Geometry: see drawing. Coordinates: mm, zero at the bounding-box minimum. Coordinates: 2 decimals unless noted, no trailing zeros. Write each loop counter-clockwise with the first axis right and the second up, starting at its lowest first coordinate (ties: lowest second). Pieces come first, ordered by that corner, then holes.
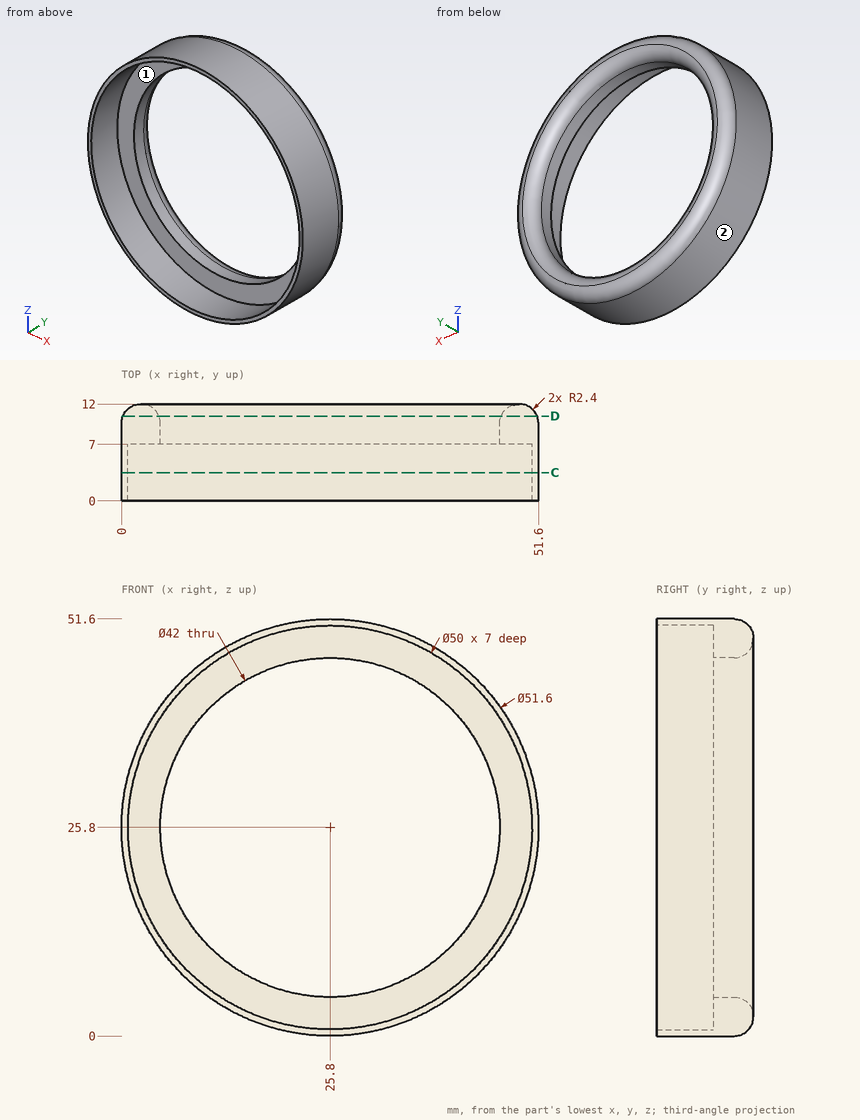
Item 1: Pull-direction query (Z, two-part tool) for the marked faces 1 and 2; classes: released by +Z, released by -Z, zero draft, split by the parting line, or undercut.
Derived:
face 1: undercut
face 2: split by the parting line
Item 2: Material intervals for probe 1 along X at (y, z) = (3.5, 25.8); probe 2 along X at (y, z) = (9, 25.8); probe 3 along Z at (x, y) = (7, 7.5), sorted ascending.
Derived:
probe 1: x = 0 to 0.8, 50.8 to 51.6
probe 2: x = 0 to 4.8, 46.8 to 51.6
probe 3: z = 8.13 to 16.44, 35.16 to 43.47
Item 3: Section C-C, the plane y = 3.5. Output: boundary loops of the cut face in (x, z), plus the area to 3 significant figures.
Derived:
outline: circle Ø51.6 at (25.8, 25.8); hole circle Ø50 at (25.8, 25.8)
area: 128 mm2
Item 4: Section D-D, the plane y = 10.5. Output: boundary loops of the cut face in (x, z) (3 decimals).
Derived:
outline: circle Ø51.25 at (25.8, 25.8); hole circle Ø42.35 at (25.8, 25.8)
Item 5: Pin query (flat end, axial travel): pin 1 (4 mm diameter, centred on x = 6, z = 31.5, fed in from +Y); pin 2 (3 mm diameter, centred on y = 3.5, z = 8, fed in from -X); pin 3 (5 mm diameter, centred on x = 15.5, y = 4.5, fed in from +Z). Return the tip coordinate at first contact, or that it passes through.
Derived:
pin 1: stops at y = 11.86
pin 2: stops at x = 5.8
pin 3: stops at z = 50.39
